from build123d import *

# Parameters (mm, degrees)
F0_W          = 25.4
F0_H          = 25.4
F1_DEPTH      = 25.4
F2_T1_DEPTH   = 88.9
F3_R          = 2.54
F4_DEPTH      = 7.62
F5_R          = 5.08
F6_DEPTH      = 5.08
F7_SIZE       = 5.07999
F8_W          = 7.62
F8_H          = 12.7
F9_DEPTH      = 25.4
F10_T1_DEPTH  = 50.8
F10_T3_DEPTH  = 50.8
F10_T5_DEPTH  = 7.62
F10_T7_DEPTH  = 12.7
F10_T13_DEPTH = 20.32
F10_T18_DEPTH = 25.4
F10_T26_DEPTH = 20.32
F10_T30_DEPTH = 25.4
F10_T38_DEPTH = 25.4
F10_T43_DEPTH = 20.32
F10_T51_DEPTH = 20.32
F10_T55_DEPTH = 25.4


# Not quite as in the source:
# - a fillet or chamfer that OpenCascade refuses, or shapes differently, is made with other operations: its cross-section is extruded or revolved along the edge and cut away or added
# - a fillet or chamfer is up to 0.001 mm smaller than in the source, because OpenCascade refuses the exact size


with BuildPart() as f1:
    # F0 (on Top) → F1 (new body)
    with BuildSketch(Plane.XY):
        with Locations((12.7, 12.7)):
            Rectangle(F0_W, F0_H)
    extrude(amount=F1_DEPTH)

    # F2: fillet of radius 12.7 on 2 edges, made by hand

    # F2_s2 → F2_t1 (cut)
    with BuildSketch(Plane.XY.offset(-31.75)):
        with BuildLine():
            ThreePointArc((0, 12.7), (3.7197438789, 3.7197438789), (12.7, 0))
            Line((12.7, 0), (0, 0))
            Line((0, 0), (0, 12.7))
        make_face()
        with BuildLine():
            ThreePointArc((12.7, 0), (21.6802561211, 3.7197438789), (25.4, 12.7))
            Line((25.4, 12.7), (25.4, 0))
            Line((25.4, 0), (12.7, 0))
        make_face()
    extrude(amount=F2_T1_DEPTH, mode=Mode.SUBTRACT)

    # F3 (on face) → F4 (join)
    with BuildSketch(Plane.XY.offset(25.4)):
        with Locations((12.7, 12.7)):
            Circle(F3_R)
    extrude(amount=F4_DEPTH)

    # F5 (on face) → F6 (join)
    with BuildSketch(Plane.XY.offset(33.02)):
        with Locations((12.7, 12.7)):
            Circle(F5_R)
    extrude(amount=F6_DEPTH)

    # F7 (size 5.08 in the source; OpenCascade refuses exactly that, so slightly less here)
    f7_edges = [f1.edges().sort_by_distance(p)[0] for p in [
        (7.62, 12.7, 38.1),
    ]]
    chamfer(f7_edges, length=F7_SIZE)

    # F8 (on face) → F9 (cut)
    with BuildSketch(Plane(origin=(0, 25.4, 0), x_dir=(-1, 0, 0), z_dir=(0, 1, 0))):
        with Locations((-16.51, 13.97)):
            Rectangle(F8_W, F8_H)
    extrude(amount=-F9_DEPTH, mode=Mode.SUBTRACT)

    # F10: fillet of radius 5.08 on 8 edges, made by hand

    # F10_s2 → F10_t1 (cut)
    with BuildSketch(Plane.XY.offset(-12.7)):
        with BuildLine():
            ThreePointArc((20.32, 25.4), (23.9121024484, 23.9121024484), (25.4, 20.32))
            Line((25.4, 20.32), (25.4, 25.4))
            Line((25.4, 25.4), (20.32, 25.4))
        make_face()
        with BuildLine():
            ThreePointArc((5.08, 25.4), (1.4878975516, 23.9121024484), (0, 20.32))
            Line((0, 20.32), (0, 25.4))
            Line((0, 25.4), (5.08, 25.4))
        make_face()
    extrude(amount=F10_T1_DEPTH, mode=Mode.SUBTRACT)

    # F10_s4 → F10_t3 (cut)
    with BuildSketch(Plane.YZ.offset(-12.7)):
        with BuildLine():
            ThreePointArc((25.4, 5.08), (23.9121024484, 1.4878975516), (20.32, 0))
            Line((20.32, 0), (25.4, 0))
            Line((25.4, 0), (25.4, 5.08))
        make_face()
        with BuildLine():
            ThreePointArc((20.32, 25.4), (23.9121024484, 23.9121024484), (25.4, 20.32))
            Line((25.4, 20.32), (25.4, 25.4))
            Line((25.4, 25.4), (20.32, 25.4))
        make_face()
    extrude(amount=F10_T3_DEPTH, mode=Mode.SUBTRACT)

    # F10_s6 → F10_t5 (cut)
    with BuildSketch(Plane.YZ.offset(12.7)):
        with BuildLine():
            ThreePointArc((25.4, 2.54), (23.9121024484, 6.1321024484), (20.32, 7.62))
            Line((20.32, 7.62), (25.4, 7.62))
            Line((25.4, 7.62), (25.4, 2.54))
        make_face()
        with BuildLine():
            ThreePointArc((25.4, 25.4), (23.9121024484, 21.8078975516), (20.32, 20.32))
            Line((20.32, 20.32), (25.4, 20.32))
            Line((25.4, 20.32), (25.4, 25.4))
        make_face()
    extrude(amount=F10_T5_DEPTH, mode=Mode.SUBTRACT)

    # F10_s8 → F10_t7 (cut)
    with BuildSketch(Plane.XY.offset(7.62)):
        with BuildLine():
            ThreePointArc((25.4, 25.4), (21.8078975516, 23.9121024484), (20.32, 20.32))
            Line((20.32, 20.32), (20.32, 25.4))
            Line((20.32, 25.4), (25.4, 25.4))
        make_face()
        with BuildLine():
            ThreePointArc((7.62, 25.4), (11.2121024484, 23.9121024484), (12.7, 20.32))
            Line((12.7, 20.32), (12.7, 25.4))
            Line((12.7, 25.4), (7.62, 25.4))
        make_face()
    extrude(amount=F10_T7_DEPTH, mode=Mode.SUBTRACT)


with BuildPart() as f10_tool11:
    # F10_s12 → F10_t13 (new body)
    with BuildSketch(Plane.YZ.offset(33.02)):
        with BuildLine():
            ThreePointArc((25.4, 2.54), (23.9121024484, 6.1321024484), (20.32, 7.62))
            Line((20.32, 7.62), (25.4, 7.62))
            Line((25.4, 7.62), (25.4, 2.54))
        make_face()
    extrude(amount=-F10_T13_DEPTH)

    split(bisect_by=Plane.YZ.offset(25.4), keep=Keep.BOTTOM)

    split(bisect_by=Plane.YZ.offset(20.32), keep=Keep.TOP)


with BuildPart() as f10_tool16:
    # F10_s17 → F10_t18 (new body)
    with BuildSketch(Plane.XY.offset(20.32)):
        with BuildLine():
            ThreePointArc((25.4, 25.4), (21.8078975516, 23.9121024484), (20.32, 20.32))
            Line((20.32, 20.32), (20.32, 25.4))
            Line((20.32, 25.4), (25.4, 25.4))
        make_face()
    extrude(amount=-F10_T18_DEPTH)

    split(bisect_by=Plane.XY, keep=Keep.TOP)

    split(bisect_by=Plane.XY.offset(7.62), keep=Keep.BOTTOM)


with BuildPart() as f10_tool11_1:
    add(f10_tool11.part)

    # F10_t21: intersect F10_tool16
    add(f10_tool16.part, mode=Mode.INTERSECT)


with BuildPart() as f1_1:
    add(f1.part)

    # F10_t9: cut F10_tool11
    add(f10_tool11_1.part, mode=Mode.SUBTRACT)


with BuildPart() as f10_tool24:
    # F10_s25 → F10_t26 (new body)
    with BuildSketch(Plane.YZ.offset(20.32)):
        with BuildLine():
            ThreePointArc((25.4, 2.54), (23.9121024484, 6.1321024484), (20.32, 7.62))
            Line((20.32, 7.62), (25.4, 7.62))
            Line((25.4, 7.62), (25.4, 2.54))
        make_face()
    extrude(amount=-F10_T26_DEPTH)

    split(bisect_by=Plane.YZ.offset(12.7), keep=Keep.BOTTOM)


with BuildPart() as f10_tool28:
    # F10_s29 → F10_t30 (new body)
    with BuildSketch(Plane.XY.offset(-5.08)):
        with BuildLine():
            ThreePointArc((7.62, 25.4), (11.2121024484, 23.9121024484), (12.7, 20.32))
            Line((12.7, 20.32), (12.7, 25.4))
            Line((12.7, 25.4), (7.62, 25.4))
        make_face()
    extrude(amount=F10_T30_DEPTH)

    split(bisect_by=Plane.XY, keep=Keep.TOP)

    split(bisect_by=Plane.XY.offset(7.62), keep=Keep.BOTTOM)


with BuildPart() as f10_tool24_1:
    add(f10_tool24.part)

    # F10_t33: intersect F10_tool28
    add(f10_tool28.part, mode=Mode.INTERSECT)


with BuildPart() as f1_2:
    add(f1_1.part)

    # F10_t22: cut F10_tool24
    add(f10_tool24_1.part, mode=Mode.SUBTRACT)


with BuildPart() as f10_tool36:
    # F10_s37 → F10_t38 (new body)
    with BuildSketch(Plane.XY.offset(33.02)):
        with BuildLine():
            ThreePointArc((25.4, 25.4), (21.8078975516, 23.9121024484), (20.32, 20.32))
            Line((20.32, 20.32), (20.32, 25.4))
            Line((20.32, 25.4), (25.4, 25.4))
        make_face()
    extrude(amount=-F10_T38_DEPTH)

    split(bisect_by=Plane.XY.offset(25.4), keep=Keep.BOTTOM)

    split(bisect_by=Plane.XY.offset(20.32), keep=Keep.TOP)


with BuildPart() as f10_tool41:
    # F10_s42 → F10_t43 (new body)
    with BuildSketch(Plane.YZ.offset(12.7)):
        with BuildLine():
            ThreePointArc((25.4, 25.4), (23.9121024484, 21.8078975516), (20.32, 20.32))
            Line((20.32, 20.32), (25.4, 20.32))
            Line((25.4, 20.32), (25.4, 25.4))
        make_face()
    extrude(amount=F10_T43_DEPTH)

    split(bisect_by=Plane.YZ.offset(25.4), keep=Keep.BOTTOM)

    split(bisect_by=Plane.YZ.offset(20.32), keep=Keep.TOP)


with BuildPart() as f10_tool36_1:
    add(f10_tool36.part)

    # F10_t46: intersect F10_tool41
    add(f10_tool41.part, mode=Mode.INTERSECT)


with BuildPart() as f1_3:
    add(f1_2.part)

    # F10_t34: cut F10_tool36
    add(f10_tool36_1.part, mode=Mode.SUBTRACT)


with BuildPart() as f10_tool49:
    # F10_s50 → F10_t51 (new body)
    with BuildSketch(Plane.YZ):
        with BuildLine():
            ThreePointArc((25.4, 25.4), (23.9121024484, 21.8078975516), (20.32, 20.32))
            Line((20.32, 20.32), (25.4, 20.32))
            Line((25.4, 20.32), (25.4, 25.4))
        make_face()
    extrude(amount=F10_T51_DEPTH)

    split(bisect_by=Plane.YZ.offset(12.7), keep=Keep.BOTTOM)


with BuildPart() as f10_tool53:
    # F10_s54 → F10_t55 (new body)
    with BuildSketch(Plane.XY.offset(7.62)):
        with BuildLine():
            ThreePointArc((7.62, 25.4), (11.2121024484, 23.9121024484), (12.7, 20.32))
            Line((12.7, 20.32), (12.7, 25.4))
            Line((12.7, 25.4), (7.62, 25.4))
        make_face()
    extrude(amount=F10_T55_DEPTH)

    split(bisect_by=Plane.XY.offset(25.4), keep=Keep.BOTTOM)

    split(bisect_by=Plane.XY.offset(20.32), keep=Keep.TOP)


with BuildPart() as f10_tool49_1:
    add(f10_tool49.part)

    # F10_t58: intersect F10_tool53
    add(f10_tool53.part, mode=Mode.INTERSECT)


with BuildPart() as f1_4:
    add(f1_3.part)

    # F10_t47: cut F10_tool49
    add(f10_tool49_1.part, mode=Mode.SUBTRACT)


solid = f1_4.part
The model under review builds one solid part; all positions refer to its coordinate system, in mm. A direction names the side the tool comes from. Coordinates: 2 decimals unless noted, no trailing zeros. Loops run counter-clockwise (first coordinate to the right, second up) from the corner with the lowest first, then second, coordinate; pieces in that order, holes last. Notation, with made-up numbers: M 25.25,1 L 51.25,1 A18 cw 51.25,22 Z; hole C 6,-33 d2. An arc over 180 degrees is marked long. Put each result on its own line as item: value. Start each with the question number.
Q1. Add section A-A (x = 18.5). Write out the cut boundary in (y, z), and give its area (3 significant figures).
Q2. For faces 5 (the flat face through (10, 12, 33.02)), 6 (the cylindrical face through (1.528, 23.951, 12.522)), 7 (the cylindrical face through (16, 23.5, 6.5)), 8 (the flat face through (17, 10, 20.32)), 9 (the cylindrical face through (12.52, 23.28, 0.95)), list the 3-axis set-ups (+Z, -Z, +X, -X, +Y, -Y) from which the entire face can be reached by the end or side of a thin tool; tool diameter is ignored.
Q3. Add section B-B (z = 7). Write out the cut boundary in (x, y).
Q4. The part is to be moulded in two halves that separate along X. For faces 1 (the flat face through (20.32, 11, 14)), 2 (the flat face through (6, 25.4, 13)), 3 (the flat face through (25.4, 16, 13)), 4 (the cylindrical face through (16.421, 23.383, 21.348)), say which applies: +X half, -X half, draft (parallel to the pull), parting line (faces both ways), or undercut.
Q5. Wall thickness on line 1 (X direction, y = 17.5, z = 15); line 2 (Z direction, x = 11, y = 2.5); line 3 (X direction, y = 22.25, z = 11): over which ranges is each line inside the solid? List them lowest first.
Q6. Add section C-C (y = 17). Count the separate pieces of the cut face and the enclosed holes in it, and give its area (3 significant figures).
Q7. Clearance check with flat-ended pins moving along their axes: pin 1 (4 mm diameter, centred on x = 14, z = 30, fed in from -Y); pin 2 (2 mm diameter, centred on y = 23, z = 11.5, fed in from +X); pin 3 (5 mm diameter, centred on x = 17, z = 7.5, fed in from +Y); pin 4 (1 mm diameter, centred on y = 9.5, z = 28.5, fed in from -X). State where each tip first meets the part, or that it passes through.
Q8. Add section D-D (z = 21). Write out the cut boundary in (x, y), and give its area (4 significant figures).
Answers:
1. outline: M 1.4,0 L 20.32,0 A5.08 ccw 25.24,3.81 A5.08 ccw 20.32,7.62 L 1.4,7.62 Z; M 1.4,20.32 L 20.32,20.32 A5.08 ccw 24.72,22.86 A5.08 ccw 20.32,25.4 L 1.4,25.4 Z
1. area: 284 mm^2
2. face 5: none
2. face 6: +Z, -Z, -X, +Y
2. face 7: +Y
2. face 8: +Y, -Y
2. face 9: -Z, +X, -X, +Y
3. outline: M 0,12.7 A12.7 ccw 25.4,12.7 L 25.4,20.32 A5.08 ccw 22.86,24.72 A5.08 ccw 20.94,22.75 L 12.08,22.75 A5.08 ccw 7.62,25.4 L 5.08,25.4 A5.08 ccw 0,20.32 Z
4. face 1: undercut
4. face 2: draft
4. face 3: +X half
4. face 4: undercut
5. line 1: x = 0 to 12.7, 20.32 to 25.4
5. line 2: z = 0 to 25.4
5. line 3: x = 0.38 to 12.32, 20.7 to 25.02
6. separate pieces: 2
6. enclosed holes: 1
6. area: 551 mm^2
7. pin 1: stops at y = 10.16
7. pin 2: stops at x = 25.11
7. pin 3: stops at y = 24.76
7. pin 4: passes through
8. outline: M 0,12.7 A12.7 ccw 25.4,12.7 L 25.4,20.32 A5.08 ccw 22.86,24.72 A5.08 ccw 21,22.86 L 12.02,22.86 A5.08 ccw 8.3,25.35 L 4.4,25.35 A5.08 ccw 0,20.32 Z
8. area: 536.5 mm^2
